```python
from build123d import *

# Parameters (mm, degrees)
BOSS_EXTRUDE1_DEPTH = 1.75
SKETCH4_W           = 1
SKETCH4_H           = 34
SKETCH4_W_2         = 19.9
SKETCH4_H_2         = 1.5
BOSS_EXTRUDE3_DEPTH = 4
SKETCH7_W           = 6
SKETCH7_H           = 0.5
BOSS_EXTRUDE5_DEPTH = 10
SKETCH9_W           = 6
SKETCH9_H           = 0.5
BOSS_EXTRUDE6_DEPTH = 10


with BuildPart() as part:
    # Sketch2 → Boss-Extrude1 (new body)
    with BuildSketch(Plane(origin=(0, 0, 0), x_dir=(1, 0, 0), z_dir=(0, 1, 0))):
        Polygon((0, 14.85), (0, 17), (-10, 17), (-10, 0), (-3, 0), (-3, 0.85), (0, 0.85), (0, 1.45), (-3, 1.45), (-3, 11.55), (0, 11.55), (0, 12.15), (-3, 12.15), (-3, 14.85), align=None)
        Polygon((-3, 0), (-10, 0), (-10, -17), (0, -17), (0, -1.85), (-3, -1.85), align=None)
        Polygon((10, -17), (10, 0), (3, 0), (3, -1.85), (0, -1.85), (0, -17), align=None)
        Polygon((10, 17), (0, 17), (0, 14.85), (3, 14.85), (3, 12.15), (0, 12.15), (0, 11.55), (3, 11.55), (3, 1.45), (0, 1.45), (0, 0.85), (3, 0.85), (3, 0), (10, 0), align=None)
    extrude(amount=BOSS_EXTRUDE1_DEPTH)

    # Sketch4 → Boss-Extrude3 (add)
    with BuildSketch(Plane(origin=(0, 0, 0), x_dir=(1, 0, 0), z_dir=(0, 1, 0))):
        with Locations((-10.5, 0)):
            Rectangle(SKETCH4_W, SKETCH4_H)
        with Locations((10.5, 0)):
            Rectangle(SKETCH4_W, SKETCH4_H)
        with Locations((0, 17.75)):
            Rectangle(SKETCH4_W_2, SKETCH4_H_2)
        with Locations((0, -17.75)):
            Rectangle(SKETCH4_W_2, SKETCH4_H_2)
    extrude(amount=BOSS_EXTRUDE3_DEPTH)

    # Sketch7 → Boss-Extrude5 (add)
    with BuildSketch(Plane.ZY.offset(11)):
        with Locations((-6.5, 0.25)):
            Rectangle(SKETCH7_W, SKETCH7_H)
    extrude(amount=BOSS_EXTRUDE5_DEPTH)

    # Sketch9 → Boss-Extrude6 (add)
    with BuildSketch(Plane(origin=(11, 0, 0), x_dir=(0, 0, -1), z_dir=(1, 0, 0))):
        with Locations((6.5, 0.25)):
            Rectangle(SKETCH9_W, SKETCH9_H)
    extrude(amount=BOSS_EXTRUDE6_DEPTH)


solid = part.part
```
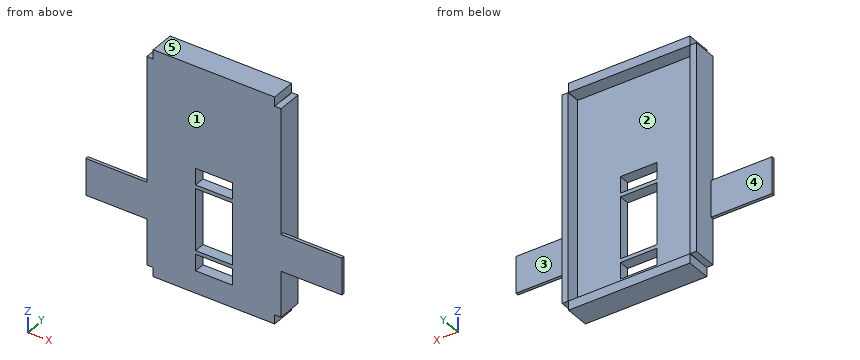
Read the model definition and answer for the solid it produces. Units are mm, in the model's axes. Face numbers are marked on the shaded views. A direction names the side the tool comes from. Round coordinates to 2 decimals unless told otherwise and drop trailing zeros. Write each loop counter-clockwise with the first axis right and the second up, starting at its lowest first coordinate (ties: lowest second). Pieces come first, ordered by that corner, then holes. Notation, with made-up numbers: (77, 89.5) - (109, 89.5) arc R20 cw to (109, 121.5) - close; hole circle Ø2 at (62, 87). An arc over 180 degrees is marked (long way). One line per item, written item: value.
Q1. Find section A-A (z = -3). Determine the outline of the cut face in (x, y).
The answers:
outline: (-11, 0) - (-3, 0) - (-3, 1.75) - (-10, 1.75) - (-10, 4) - (-11, 4) - close; (3, 0) - (11, 0) - (11, 4) - (10, 4) - (10, 1.75) - (3, 1.75) - close
Q2. Which of the six approach directions +Z, -Z, +X, -X, +Y, -Y give full straight-line access (tool end or side, diameter ignored) to the marked faces 3, 4 and 5?
The answers:
face 3: +Z, -Z, +X, +Y
face 4: +Z, -Z, -X, +Y
face 5: +Z, +X, -X, +Y, -Y
Q3. For a pull along X with two mould halves and no side action, classify the marked faces 1 and 2 as pulls with the +X half, pulls with the -X half, needs draft (parallel to the pull), parting line crosses it, or undercut.
The answers:
face 1: needs draft
face 2: undercut
Q4. Find section D-D (z = -8). Determine the outline of the cut face in (x, y).
The answers:
outline: (-21, 0) - (-3, 0) - (-3, 1.75) - (-10, 1.75) - (-10, 4) - (-11, 4) - (-11, 0.5) - (-21, 0.5) - close; (3, 0) - (21, 0) - (21, 0.5) - (11, 0.5) - (11, 4) - (10, 4) - (10, 1.75) - (3, 1.75) - close
Q5. Each of these flat-tipped pins is pushed along its axis until it touches: P1, Ø6, axis at x = -4.5, z = -7, coming from the +Y side; P2, Ø1.9, axis at y = 0.5, z = 0.5, coming from the +X side; P3, Ø8, axis at x = 9, z = -14, coming from the +Y side; P4, Ø2, axis at x = -14.5, y = 1, coming from the -Z side. Where does it stop, or does it pass through?
The answers:
P1: stops at y = 1.75
P2: stops at x = 11
P3: stops at y = 4
P4: stops at z = -9.5
Q6. Find section C-C (y = 2.65). Determine the outline of the cut face in (x, z), and give its area (3 significant figures).
The answers:
outline: (-11, -17) - (-10, -17) - (-10, 17) - (-11, 17) - close; (-9.95, -18.5) - (9.95, -18.5) - (9.95, -17) - (-9.95, -17) - close; (-9.95, 17) - (9.95, 17) - (9.95, 18.5) - (-9.95, 18.5) - close; (10, -17) - (11, -17) - (11, 17) - (10, 17) - close
area: 128 mm2
Q7. Straight lines are drawn through the part: line 1 (Z direction, x = 2, y = 0.6); line 2 (X direction, y = 2.4, z = 3); line 3 (Z direction, x = -4, y = 3.2). For each, find the intervals that lie inside material, in ascending order. Write a range as from..to.
The answers:
line 1: z = -18.5..-14.85, -12.15..-11.55, -1.45..-0.85, 1.85..18.5
line 2: x = -11..-10, 10..11
line 3: z = -18.5..-17, 17..18.5
Q8. Find section B-B (x = -1.5). Determine the outline of the cut face in (y, z), and give its area (3 significant figures).
The answers:
outline: (0, -18.5) - (4, -18.5) - (4, -17) - (1.75, -17) - (1.75, -14.85) - (0, -14.85) - close; (0, -12.15) - (1.75, -12.15) - (1.75, -11.55) - (0, -11.55) - close; (0, -1.45) - (1.75, -1.45) - (1.75, -0.85) - (0, -0.85) - close; (0, 1.85) - (1.75, 1.85) - (1.75, 17) - (4, 17) - (4, 18.5) - (0, 18.5) - close
area: 44.4 mm2
